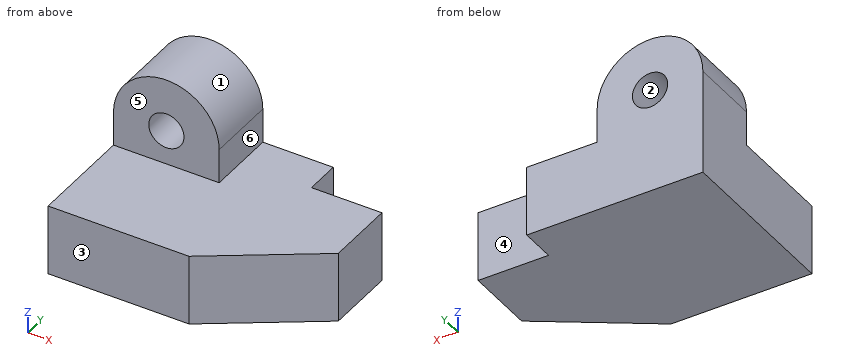
from build123d import *

# Parameters (mm, degrees)
F1_DEPTH = 20
F3_DEPTH = 20
F4_R     = 5
F5_DEPTH = 20


with BuildPart() as f1:
    # F0 (on Top) → F1 (new body)
    with BuildSketch(Plane.XY):
        Polygon((0, 50), (0, 0), (40, 0), (70, 20), (70, 40), (50, 40), (50, 50), align=None)
    extrude(amount=F1_DEPTH)

    # F2 (on face) → F3 (join)
    with BuildSketch(Plane(origin=(0, 50, 0), x_dir=(-1, 0, 0), z_dir=(0, 1, 0))):
        with BuildLine():
            Line((-3.633996, 20), (0, 20))
            Line((0, 20), (0, 29.788461))
            ThreePointArc((0, 29.788461), (-0.937816, 24.567831), (-3.633996, 20))
        make_face()
        with BuildLine():
            ThreePointArc((-26.366004, 20), (-29.062184, 24.567831), (-30, 29.788461))
            Line((-30, 29.788461), (-30, 20))
            Line((-30, 20), (-26.366004, 20))
        make_face()
        with BuildLine():
            Line((0, 0), (0, 20))
            Line((0, 20), (-3.633996, 20))
            ThreePointArc((-3.633996, 20), (-15, 14.788461), (-26.366004, 20))
            Line((-26.366004, 20), (-30, 20))
            Line((-30, 20), (-50, 20))
            Line((-50, 20), (-50, 0))
            Line((-50, 0), (0, 0))
        make_face()
        with BuildLine():
            Line((-30, 29.788461), (0, 29.788461))
            ThreePointArc((0, 29.788461), (-15, 44.788461), (-30, 29.788461))
        make_face()
        with BuildLine():
            ThreePointArc((-3.633996, 20), (-0.937816, 24.567831), (0, 29.788461))
            Line((0, 29.788461), (-30, 29.788461))
            ThreePointArc((-30, 29.788461), (-29.062184, 24.567831), (-26.366004, 20))
            Line((-26.366004, 20), (-3.633996, 20))
        make_face()
    extrude(amount=-F3_DEPTH)

    # F4 (on face) → F5 (cut, through all)
    with BuildSketch(Plane(origin=(0, 50, 0), x_dir=(-1, 0, 0), z_dir=(0, 1, 0))):
        with Locations((-15, 29.788461)):
            Circle(F4_R)
    extrude(amount=-F5_DEPTH, mode=Mode.SUBTRACT)


solid = f1.part
Here's how the part is built. I have some questions about the finished solid (model axes, mm). Face numbers are marked on the shaded views. A direction names the side the tool comes from. Coordinates: 2 decimals unless noted, no trailing zeros. Write each loop counter-clockwise with the first axis right and the second up, starting at its lowest first coordinate (ties: lowest second). Pieces come first, ordered by that corner, then holes.
1) If we section it at A-A (x = 15): List the corners of the cut face in (y, z) for me.
Filled in:
outline: (0, 0) - (50, 0) - (50, 24.79) - (30, 24.79) - (30, 20) - (0, 20) - close; (30, 34.79) - (50, 34.79) - (50, 44.79) - (30, 44.79) - close
2) If I drill on line 1 (Z direction, x = 15, y = 35); line 2 (Z direction, x = 44, y = 25); line 3 (X direction, y = 48.5, z = 9.5), over which ranges is the centre line in solid material (lowest first)?
Filled in:
line 1: z = 0 to 24.79, 34.79 to 44.79
line 2: z = 0 to 20
line 3: x = 0 to 50
3) Thinking about a two-plate mould opening in X: for the marked faces 1, 2 and 3, which applies, +X half, -X half, draft (parallel to the pull), parting line (faces both ways), or undercut?
Filled in:
face 1: parting line
face 2: undercut
face 3: draft
4) I'm going to push flat-ended pins straight in: pin 1 (12 mm diameter, centred on x = 23, z = 28, fed in from -Y); pin 2 (8 mm diameter, centred on x = 15, z = 29.79, fed in from -Y); pin 3 (11 mm diameter, centred on y = 46, z = 6.5, fed in from +X); pin 4 (15 mm diameter, centred on x = 46, y = 20, fed in from +Z). Where does each tip first touch, or does it pass through?
Filled in:
pin 1: stops at y = 30
pin 2: passes through
pin 3: stops at x = 50
pin 4: stops at z = 20
5) If we section it at D-D (z = 33.5): List the corners of the cut face in (x, y) for me, plus the area to 3 significant figures.
Filled in:
outline: (0.47, 30) - (11.65, 30) - (11.65, 50) - (0.47, 50) - close; (18.35, 30) - (29.53, 30) - (29.53, 50) - (18.35, 50) - close
area: 447 mm2
6) If we section it at C-C (y = 29): List the corners of the cut face in (x, z) for me.
Filled in:
outline: (0, 0) - (70, 0) - (70, 20) - (0, 20) - close
7) If we section it at B-B (z = 10): List the corners of the cut face in (x, y) for me.
Filled in:
outline: (0, 0) - (40, 0) - (70, 20) - (70, 40) - (50, 40) - (50, 50) - (0, 50) - close
8) Which directions (+Z, -Z, +X, -X, +Y, -Y) give clear straight access to the entire face, cutting with the end or side of a thin tool? Please do the marked faces 4, 5 and 6.
Filled in:
face 4: +Z, -Z, +X, +Y
face 5: +Z, +X, -X, -Y
face 6: +Z, +X, +Y, -Y
